from build123d import *

# Parameters (mm, degrees)
ESQUISSE1_R             = 3
BOSS_EXTRU_1_DEPTH      = 4
ESQUISSE2_R             = 2
BOSS_EXTRU_2_DEPTH      = 20
CHANFREIN1_SIZE         = 0.25
ENL_V_START             = -1.5
ENL_V_MAT_EXTRU_1_DEPTH = 1.5
BOSS_EXTRU_3_START      = 1
ESQUISSE4_R             = 2
BOSS_EXTRU_3_DEPTH      = 1
ESQUISSE5_R             = 1.875
BOSS_EXTRU_4_DEPTH      = 14
CHANFREIN2_SIZE         = 1


with BuildPart() as part:
    # Esquisse1 → Boss.-Extru.1 (new body)
    with BuildSketch(Plane(origin=(0, 0, 0), x_dir=(1, 0, 0), z_dir=(0, 1, 0))):
        with Locations(Location((0, 0, 0), (0, 0, 270))):
            Circle(ESQUISSE1_R)
    extrude(amount=BOSS_EXTRU_1_DEPTH)

    # Esquisse2 → Boss.-Extru.2 (add)
    with BuildSketch(Plane(origin=(0, 4, 0), x_dir=(1, 0, 0), z_dir=(0, 1, 0))):
        with Locations(Location((0, 0, 0), (0, 0, 270))):
            Circle(ESQUISSE2_R)
    extrude(amount=BOSS_EXTRU_2_DEPTH)

    # Chanfrein1
    chanfrein1_edges = [part.edges().sort_by_distance(p)[0] for p in [
        (0, 24, -2),
    ]]
    chamfer(chanfrein1_edges, length=CHANFREIN1_SIZE)

    # Esquisse3 → Enlèv. mat.-Extru.1 (cut)
    with BuildSketch(Plane(origin=(0, 24, 0), x_dir=(1, 0, 0), z_dir=(0, 1, 0)).offset(ENL_V_START)):
        with BuildLine():
            Line((-1.936491673, -0.5), (1.936491673, -0.5))
            ThreePointArc((1.936491673, -0.5), (2, 0), (1.936491673, 0.5))
            Line((1.936491673, 0.5), (-1.936491673, 0.5))
            ThreePointArc((-1.936491673, 0.5), (-2, 0), (-1.936491673, -0.5))
        make_face()
    extrude(amount=ENL_V_MAT_EXTRU_1_DEPTH, mode=Mode.SUBTRACT)

    # Esquisse4 → Boss.-Extru.3 (add)
    with BuildSketch(Plane.XZ.offset(BOSS_EXTRU_3_START)):
        with Locations(Location((0, 0, 0), (0, 0, 194.477512186))):
            Circle(ESQUISSE4_R)
    extrude(amount=-BOSS_EXTRU_3_DEPTH)

    # Esquisse5 → Boss.-Extru.4 (add)
    with BuildSketch(Plane.XZ.offset(1)):
        with Locations(Location((0, 0, 0), (0, 0, 270))):
            Circle(ESQUISSE5_R)
    extrude(amount=BOSS_EXTRU_4_DEPTH)

    # Chanfrein2
    chanfrein2_edges = [part.edges().sort_by_distance(p)[0] for p in [
        (0, -15, 1.875),
    ]]
    chamfer(chanfrein2_edges, length=CHANFREIN2_SIZE)


solid = part.part
Check sheet for the modelled part. Datum: model origin and axes. Units: mm. A direction names the side the tool comes from. Give positions to 0.01 mm unless a question says otherwise; leave off trailing zeros. Loops run counter-clockwise (first coordinate to the right, second up) from the corner with the lowest first, then second, coordinate; pieces in that order, holes last. Notation, with made-up numbers: M -26.5,-6.5 L -2.5,-6.5 A21 ccw -2.5,-0.5 Z; hole C -13.5,29.5 d10. An arc over 180 degrees is marked long. Answer as a JSON object with one key per item and string values. Group by question number.
Q1. Cross-section at A-A on z = 0. Record the cut outline in (x, y) (3 decimals).
Q2. Cross-section at C-C on y = 1.5. Record the cut outline in (x, z), then the cut area to 3 significant figures.
Q3. Cross-section at D-D on y = -9. Record the cut outline in (x, z) (3 decimals), then the cut area to 3 significant figures.
Q4. Cross-section at B-B on x = 0. Record the cut outline in (y, z) (3 decimals), then the cut area to 3 significant figures.
Q5. Material ranges on line 1 along Y through (x, z) = (0.8, -2.6); line 2 along Y through (x, z) = (-0.2, 0); line 3 along Z through (x, y) = (0.85, -6.5), recorded low to high. Write a range as [from, to].
Q6. Access from +Z, -Z, +X, -X, +Y, -Y to the whole of each face (thin tool, end or side, straight path). Record for faces 1 (the cylindrical face through (0.9, 1.97, 2.86)), 2 (the cylindrical face through (1.2, -0.5, 1.6)), 3 (the flat face through (0, 23, 0.5)), 4 (the cylindrical face through (-0.766, 13.737, 1.847)).
Q7. Go/stop test with flat-tipped pins: P1, Ø2, axis at x = 0.5, y = -2.5, coming from the -Z side (3 decimals); P2, Ø1, axis at x = -1.5, y = 0, coming from the +Z side; P3, Ø1, axis at y = 17, z = -0.5, coming from the -X side. Record where each tip stops, or that it passes through.
Evaluation:
{
 "1": {"outline": "M -3,0 L -2,0 L -2,-1 L -1.875,-1 L -1.875,-14 L -0.875,-15 L 0.875,-15 L 1.875,-14 L 1.875,-1 L 2,-1 L 2,0 L 3,0 L 3,4 L 2,4 L 2,22.5 L -2,22.5 L -2,4 L -3,4 Z"},
 "2": {"outline": "C 0,0 d6", "area": "28.3 mm2"},
 "3": {"outline": "C 0,0 d3.75", "area": "11.0 mm2"},
 "4": {"outline": "M -15,-0.875 L -14,-1.875 L -1,-1.875 L -1,-2 L 0,-2 L 0,-3 L 4,-3 L 4,-2 L 23.75,-2 L 24,-1.75 L 24,-0.5 L 22.5,-0.5 L 22.5,0.5 L 24,0.5 L 24,1.75 L 23.75,2 L 4,2 L 4,3 L 0,3 L 0,2 L -1,2 L -1,1.875 L -14,1.875 L -15,0.875 Z", "area": "158 mm2"},
 "5": {"line 1": "y = [0, 4]", "line 2": "y = [-15, 22.5]", "line 3": "z = [-1.67, 1.67]"},
 "6": {"face 1": "+Y, -Y", "face 2": "-Y", "face 3": "+X, -X, +Y", "face 4": "+Y"},
 "7": {"P1": "stops at z = -1.875", "P2": "stops at z = 2.83", "P3": "stops at x = -2"}
}
